Source: CAD feature listing. Evaluate the final solid. Frame: model axes, mm. A direction names the side the tool comes from. Round coordinates to 2 decimals unless told otherwise and drop trailing zeros. Return JSON: item names as keys, results as strings. Group by question number.
1) Ray query, line 1 (Y direction, x = 2, z = 0); line 2 (Y direction, x = 1.75, z = 0); line 3 (Z direction, x = 0.75, y = -1). Return the intervals inside material, ascending. Write a range as from..to.
2) Mould query, pull axis X, two halves, no side actions, for faces 1 (the cylindrical face through (3.05, 2.15, -0.68)), 2 (the flat face through (0.637, 0.382, 1.307)), 3 (the flat face through (6, 0, 0)). Classes: pulls with the +X half, pulls with the -X half, needs draft (parallel to the pull), parting line crosses it, or undercut.
3) Access query for faces 4 (the conical face through (0.64, -0.01, 1.89)), 5 (the cylindrical face through (4.92, -0.54, 2.44)), 6 (the cylindrical face through (0.18, 4.197, 1.322)). Directions: +Z, -Z, +X, -X, +Y, -Y. A direction counts if a zero-diameter tool reaches every point of the face in a straight line with its end or side. Return the directions, or none.
4) Contact query for flat-ended pins moving along their axis: P1, Ø2, axis at y = 0, z = 0.5, coming from the -X side; P2, Ø1.5, axis at x = 1.5, y = -3, coming from the +Z side. Output: stop coordinate, or through.
Autodesk Inventor part; units mm, degrees
ref_plane "Work Plane2" through (3.35, 0, 0) normal (0, 0, -1) x (1, 0, 0)
ref_plane "YZ Plane" through (0, 0, 0) normal (1, 0, 0) x (0, 1, 0)
ref_plane "XZ Plane" through (0, 0, 0) normal (0, 1, 0) x (-1, 0, 0)
sketch "Sketch1" plane through (0, 0, 0) normal (0, 0, 1) x (1, 0, 0)
  line L0 (2.05, 0) -> (6, 0)
  line L1 (6, 0) -> (6, 2.5)
  line L2 (6, 2.5) -> (4.1, 2.5)
  line L3 (4.1, 2.5) -> (3.6092, 2.2546)
  line L4 (3.6092, 2.2546) -> (2.5, 2.2546)
  line L5 (0, 4.4) -> (0, 2.21)
  line L6 (0, 2.21) -> (1.1905, 1.6164)
  line L7 (1.1905, 1.6164) -> (2.05, 0)
  line L8 (-1.2, 0) -> (7.2, 0)
  line L9 (0, -0.88) -> (0, 5.28)
  line L10 (0, 4.4) -> (0.3546, 4.4)
  line L11 (0.3546, 4.4) -> (2.5, 2.2546)
  line L12 (4.1, 2.5) -> (2.2546, 2.5) construction
  dimension "d1" = 1.9
  dimension "d2" = 5
  dimension "d3" = 4.5092
  dimension "d4" = 4.42
  dimension "d5" = 26.5
  dimension "d6" = 62
  dimension "d7" = 2.05
  dimension "d8" = 0.4908
  dimension "d12" = 8.8
  dimension "d13" = 45
  dimension "d15" = 6
  dimension "d24" = 2.5
revolve "Body" add sketch "Sketch1" angle 360 about axis through (2.05, 0, 0) along (1, 0, 0) contours L7 L6 L5 L10 L11 L4 L3 L2 L1 L0
sketch "Sketch2" plane through (0, 0, 0) normal (-1, 0, 0) x (0, 0, 1)
  line L0 (0, 2.21) -> (0, 0) construction
  line L1 (0, 0) -> (2.21, 0) construction
  arc A0 (0.663, 0) -> (0, 0.663) centre (0, 0) ccw construction
  arc A1 (0.7735, 0) -> (0, 0.7735) centre (0, 0) ccw construction
  arc A2 (2.1539, 0.495) -> (0.495, 2.1539) centre (0, 0) ccw
  line L2 (0, 0) -> (1.5627, 1.5627) construction
  line L3 (0.495, 2.1539) -> (0.3952, 0.6649)
  line L4 (2.1539, 0.495) -> (0.6649, 0.3952)
  arc A3 (0.495, 2.1539) -> (0, 2.21) centre (0, 0) ccw
  arc A4 (2.21, 0) -> (2.1539, 0.495) centre (0, 0) ccw
  line L5 (0, -6.16) -> (0, 6.16)
  line L6 (-6.16, 0) -> (6.16, 0)
  arc A5 (0.495, -2.1539) -> (2.1539, -0.495) centre (0, 0) ccw
  line L7 (0.495, -2.1539) -> (0.3952, -0.6649)
  line L8 (2.1539, -0.495) -> (0.6649, -0.3952)
  arc A6 (0, -2.21) -> (0.495, -2.1539) centre (0, 0) ccw
  arc A7 (2.1539, -0.495) -> (2.21, 0) centre (0, 0) ccw
  arc A8 (-0.495, 2.1539) -> (-2.1539, 0.495) centre (0, 0) ccw
  line L9 (-0.495, 2.1539) -> (-0.3952, 0.6649)
  line L10 (-2.1539, 0.495) -> (-0.6649, 0.3952)
  arc A9 (0, 2.21) -> (-0.495, 2.1539) centre (0, 0) ccw
  arc A10 (-2.1539, 0.495) -> (-2.21, 0) centre (0, 0) ccw
  arc A11 (-0.495, -2.1539) -> (0, -2.21) centre (0, 0) ccw
  arc A12 (-2.1539, -0.495) -> (-0.495, -2.1539) centre (0, 0) ccw
  arc A13 (-2.21, 0) -> (-2.1539, -0.495) centre (0, 0) ccw
  line L11 (-2.1539, -0.495) -> (-0.6649, -0.3952)
  line L12 (-0.495, -2.1539) -> (-0.3952, -0.6649)
  arc A14 (0.3952, 0.6649) -> (0.6649, 0.3952) centre (0.648, 0.648) ccw
  arc A15 (0.6649, -0.3952) -> (0.3952, -0.6649) centre (0.648, -0.648) ccw
  arc A16 (-0.6649, 0.3952) -> (-0.3952, 0.6649) centre (-0.648, 0.648) ccw
  arc A17 (-0.3952, -0.6649) -> (-0.6649, -0.3952) centre (-0.648, -0.648) ccw
  point P0 (1.5627, -1.5627)
  point P1 (-1.5627, 1.5627)
  point P2 (-1.5627, -1.5627)
  dimension "d17" = 1.326
  dimension "d18" = 1.547
  dimension "d19" = 4.42
  dimension "d20" = 45
  dimension "d21" = 0.495
extrude "Slot" add sketch "Sketch2" against normal up to next draft 5 contours L4 A14 L3 A2 | A5 L7 A15 L8 | L9 A16 L10 A8 | A12 L11 A17 L12
fillet "Fillet1" radius 0.198 4 edges at (0, 2.21, 0) (0, 0, -2.21) (0, -2.21, 0) (0, 0, 2.21)
thread "Thread"
chamfer "Chamfer1" distance 0.4908 distance2 0.2454 1 edges at (6, -2.5, 0) measured on face at (6, 0.6238, 0.5526)
ref_plane "Work Plane2" through (3.35, 0, 0) normal (0, 0, -1) x (1, 0, 0)
equation "\"d1\" = GEL"
equation "\"d2\" = GD"
equation "\"d3\" = BDM"
equation "\"d4\" = SDM"
equation "\"d7\" = INTI"
equation "\"d8\" = GAL"
equation "\"d12\" = KOD"
equation "\"d13\" = 0.5 * SEWI"
equation "\"d15\" = NLG"
equation "\"d24\" = KOH"
equation "\"d17\" = 0.3 * SDM"
equation "\"d18\" = 0.35 * SDM"
equation "\"d19\" = SDM"
equation "\"d21\" = 0.5 * SBR"
equation "\"d23\" = 0.2 * SBR"
equation "\"d10\" = GEL"
equation "\"d25\" = -0.5 * SPD + 0.5 * GD"
equation "\"d26\" = 0.5 * GAL"
equation "\"NLG\" = 6"
equation "\"GEL\" = 1.9"
equation "\"GAL\" = 0.61345 * PTC"
equation "\"SPD\" = NND - 1.2269 * PTC"
equation "\"KOD\" = 8.8"
equation "\"KOH\" = 2.5"
equation "\"SBR\" = 0.99"
equation "\"INTI\" = 2.05"
equation "\"SDM\" = 4.42"
equation "\"GD\" = NND"
equation "\"BDM\" = NND - GAL"
equation "\"SEWI\" = 90deg"
equation "\"d9\" = SDM"
equation "\"GUL\" = 0.61345 * PTC"
equation "\"TOA\" = 30deg"
equation "\"EPV\" = 5"
equation "\"THREADDIA\" = 5"
equation "\"RR\" = 0.5"
equation "\"PTC\" = 0.8"
equation "\"NND\" = 5"
equation "\"GD1\" = THREADDIA - 1.2269 * PTC"
properties part number "AS 1427 - M5 x 6" material "Steel, Mild"
Geometry check:
{
 "1": {"line 1": "-2.75..-0.09, 0.09..2.75", "line 2": "-3..-0.56, 0.56..3", "line 3": "-3.88..-0.35, 0.35..3.88"},
 "2": {"face 1": "undercut", "face 2": "pulls with the -X half", "face 3": "pulls with the +X half"},
 "3": {"face 4": "-X", "face 5": "+X", "face 6": "+X, -X"},
 "4": {"P1": "x = 0", "P2": "z = 2.89"}
}
